from build123d import *


# Not quite as in the source:
# - a feature names something its author has since deleted; it is built from what else it names


with BuildPart() as f1:
    # F0 (on Front) → F1 (revolve)
    with BuildSketch(Plane.XZ):
        Polygon((-78, 139.9767085075), (-70, 139.9767085075), (-48.5, 189.5767085075), (-64.9242475629, 157.222121954), align=None)
        Polygon((-74.508, -10.1073468104), (-74.508, 14.9767085075), (-70, 14.9767085075), (-70, 64.7767065075), (-70, 139.9767085075), (-78, 139.9767085075), (-74.508, 64.7767065075), (-78, -10.1073468104), align=None)
    revolve(axis=Axis((-35, 0, -12.4232914925), (0, 0, 1)))


solid = f1.part
Build history of the part. All positions in model axes, mm. A direction names the side the tool comes from. Give positions to 0.01 mm unless a question says otherwise; leave off trailing zeros. Loops run counter-clockwise (first coordinate to the right, second up) from the corner with the lowest first, then second, coordinate; pieces in that order, holes last. Notation, with made-up numbers: (-29.75, 14) -> (-8.75, 14) arc R29 ccw to (-8.75, 38) -> close; hole circle Ø2 at (11, -12). An arc over 180 degrees is marked (long way). Answer in a Markdown table with one row per item.
Item 1: Slice it at C-C on z = 143.5. Write the cut outline in (x, y), plus the area to 3 significant figures.
Findings below:
| item | result |
|---|---|
| outline | circle Ø80.66 at (-35, 0); hole circle Ø66.95 at (-35, 0) |
| area | 1,590 mm² |
Item 2: Mould opens along X. For faces 4 (the conical face through (-28.336, 30.011, 156.143)), 5 (the conical face through (-19.67, 11.76, 176.15)), 6 (the flat face through (-11, 26, 14.977)), 7 (the flat face through (-54, 35, -10.107)) say: pulls with the +X half, pulls with the -X half, needs draft (parallel to the pull), parting line crosses it, or undercut.
Findings below:
| item | result |
|---|---|
| face 4 | parting line crosses it |
| face 5 | undercut |
| face 6 | undercut |
| face 7 | needs draft |
Item 3: Slice it at B-B on y = 0. Write the cut outline in (x, z).
Findings below:
| item | result |
|---|---|
| outline | (-78, -10.11) -> (-74.51, -10.11) -> (-74.51, 14.98) -> (-70, 14.98) -> (-70, 139.98) -> (-48.5, 189.58) -> (-64.92, 157.22) -> (-78, 139.98) -> (-74.51, 64.78) -> close; (-21.5, 189.58) -> (0, 139.98) -> (0, 14.98) -> (4.51, 14.98) -> (4.51, -10.11) -> (8, -10.11) -> (4.51, 64.78) -> (8, 139.98) -> (-5.08, 157.22) -> close |
Item 4: Slice it at A-A on x = -35. Write the cut outline in (y, z), plus the area to 3 significant figures.
Findings below:
| item | result |
|---|---|
| outline | (-43, -10.11) -> (-39.51, -10.11) -> (-39.51, 14.98) -> (-35, 14.98) -> (-35, 139.98) -> (-13.5, 189.58) -> (-29.92, 157.22) -> (-43, 139.98) -> (-39.51, 64.78) -> close; (13.5, 189.58) -> (35, 139.98) -> (35, 14.98) -> (39.51, 14.98) -> (39.51, -10.11) -> (43, -10.11) -> (39.51, 64.78) -> (43, 139.98) -> (29.92, 157.22) -> close |
| area | 1,910 mm² |
Item 5: Probe line 1 along X through (y, z) = (0, 64.5); line 2 along Y through (x, z) = (-51, 76); line 3 along X through (y, z) = (0, 82.5). List the from-to ranges inside material, lowest first. Write a range as [from, to].
Findings below:
| item | result |
|---|---|
| line 1 | x = [-74.52, -70], [0, 4.52] |
| line 2 | y = [-36.69, -31.13], [31.13, 36.69] |
| line 3 | x = [-75.33, -70], [0, 5.33] |
Item 6: Slice it at D-D on z = 37. Write the cut outline in (x, y), plus the area to 3 significant figures.
Findings below:
| item | result |
|---|---|
| outline | circle Ø81.61 at (-35, 0); hole circle Ø70 at (-35, 0) |
| area | 1,380 mm² |
Item 7: Tool access for faces 1 (the conical face through (-74.326, -12.384, 101.85)), 2 (the conical face through (-43.4, 16.1, 180.4)), 3 (the cylindrical face through (-5.88, -26.7, 2.61)): list every direction of +Z, -Z, +X, -X, +Y, -Y with a clear straight run to the whole face (end or side of a thin tool).
Findings below:
| item | result |
|---|---|
| face 1 | none |
| face 2 | +Z |
| face 3 | -Z |
Item 8: Flat gauge pins, fed straight in: P1, Ø1.5, axis at y = 28.5, z = 94, coming from the +X side; P2, Ø1.5, axis at x = -51, z = 22, coming from the +Y side; P3, Ø1.5, axis at x = -10.5, z = 116.5, coming from the -Y side. Where does each tip first touch, or does it go through?
Findings below:
| item | result |
|---|---|
| P1 | stops at x = -5 |
| P2 | stops at y = 38.6 |
| P3 | stops at y = -34.53 |
